Verification items for the finished model (mm, model axes). Face numbers are marked on the shaded views. A direction names the side the tool comes from. Coordinates: 2 decimals unless noted, no trailing zeros. Order: outer loops, then holes, each group sorted by start corner. A loop starts at its lowest first (then second) coordinate and runs counter-clockwise, first axis right, second up. Notation, with made-up numbers: (-37.5, 69.5) -> (-27.5, 69.5) arc R26 ccw to (-27.5, 104.5) -> close; hole circle Ø8 at (57.25, -33). An arc over 180 degrees is marked (long way). Write each question's results on one line, items separated by ' | '. Start each with the question number.
(1) Go/stop test with flat-tipped pins: pin 1 (5 mm diameter, centred on x = 16.16, y = 28, fed in from +Z); pin 2 (11.5 mm diameter, centred on x = -35.5, y = -2, fed in from +Z); pin 3 (9 mm diameter, centred on y = 9.5, z = 20.5, fed in from -X); pin 4 (1 mm diameter, centred on x = -15.5, y = 27.5, fed in from -Z). Record where each tip stops, or that it passes through.
(2) Draft check along X on the marked faces 5, 6, 7 and 8. Enter one of: +X half, -X half, draft (parallel to the pull), parting line (faces both ways), or undercut.
(3) Cross-section at C-C on z = 26.5. Enter the section's corners in (x, y), and give its area (3 significant figures).
(4) Thickness scan on probe 1 along X at (y, z) = (0, 6.75); probe 2 along X at (y, z) = (0, 11.95); probe 3 along Y at (x, z) = (-3, 22). Record the ranges inside material, lowest first. Write a range as [from, to].
(5) Cross-section at A-A on x = 0. Enter the section's corners in (y, z).
(6) Cross-section at D-D on x = -10. Give the number of separate pieces and of enclosed holes in the cut face, and give its area (3 significant figures).
(7) Cross-section at B-B on z = 22. Enter the section's corners in (x, y), and give its area (3 significant figures).
(8) Set-up check for the marked faces 1, 2, 3 and 4: record each of +Z, -Z, +X, -X, +Y, -Y from which the full face is reachable in a straight line by a thin tool's end or side.
```python
from build123d import *

# Parameters (mm, degrees)
SKETCH1_R                                     = 39.5
SKETCH1_R_2                                   = 28.5
BOSS_EXTRUDE1_DEPTH                           = 11
SKETCH2_R                                     = 39.5
BOSS_EXTRUDE2_DEPTH                           = 20
CUT_EXTRUDE3_START                            = -27
CUT_EXTRUDE3_DEPTH                            = 27
CUT_EXTRUDE4_START                            = -18
CUT_EXTRUDE4_DEPTH                            = 18
CBORE_FOR_M3_HEX_HEAD_MACHINE_SCREW1_AT_COUNT = 2
CBORE_FOR_M3_HEX_HEAD_MACHINE_SCREW1_AT_PITCH = 68
CBORE_FOR_M3_HEX_HEAD_MACHINE_SCREW1_2_COUNT  = 2
CBORE_FOR_M3_HEX_HEAD_MACHINE_SCREW1_2_PITCH  = 58.889727457
CBORE_FOR_M3_HEX_HEAD_MACHINE_SCREW1_3_COUNT  = 2
CBORE_FOR_M3_HEX_HEAD_MACHINE_SCREW1_3_PITCH  = 34
FILLET2_R                                     = 2
CBORE_FOR_M3_HEX_HEAD_MACHINE_SCREW2_AT_COUNT = 2
CBORE_FOR_M3_HEX_HEAD_MACHINE_SCREW2_AT_PITCH = 32.326095378
CUT_EXTRUDE5_DEPTH                            = 82.740442866
CUT_EXTRUDE5_DEPTH_BACK                       = 82.740442866
SKETCH10_R                                    = 2
FILLET5_R                                     = 5
FILLET4_R                                     = 5
FILLET6_R                                     = 1
FILLET7_R                                     = 10


with BuildPart() as part:
    # Sketch1 → Boss-Extrude1 (new body)
    with BuildSketch(Plane.XY):
        Circle(SKETCH1_R)
        Circle(SKETCH1_R_2, mode=Mode.SUBTRACT)
    extrude(amount=BOSS_EXTRUDE1_DEPTH)

    # Sketch2 → Boss-Extrude2 (add)
    with BuildSketch(Plane.XY.offset(11)):
        Circle(SKETCH2_R)
    extrude(amount=BOSS_EXTRUDE2_DEPTH)

    # Sketch3 → Cut-Extrude3 (cut)
    with BuildSketch(Plane.XY.offset(31).offset(CUT_EXTRUDE3_START)):
        with BuildLine():
            ThreePointArc((-32.806249405, -22), (0, -39.5), (32.806249405, -22))
            Line((32.806249405, -22), (-32.806249405, -22))
        make_face()
    extrude(amount=CUT_EXTRUDE3_DEPTH, mode=Mode.SUBTRACT)

    # Sketch4 → Cut-Extrude4 (cut)
    with BuildSketch(Plane.XY.offset(31).offset(CUT_EXTRUDE4_START)):
        with BuildLine():
            Line((-32.806249405, -22), (-25, -22))
            Line((-25, -22), (-25, 30.581857367))
            ThreePointArc((-25, 30.581857367), (-39.071774321, 5.800556129), (-32.806249405, -22))
        make_face()
        with BuildLine():
            Line((25, 30.581857367), (25, -22))
            Line((25, -22), (32.806249405, -22))
            ThreePointArc((32.806249405, -22), (39.071774321, 5.800556129), (25, 30.581857367))
        make_face()
    extrude(amount=CUT_EXTRUDE4_DEPTH, mode=Mode.SUBTRACT)

    # Sketch6 → CBORE for M3 Hex Head Machine Screw1 (revolve, cut)
    with BuildSketch(Plane(origin=(-34, 0, 13), x_dir=(0, -1, 0), z_dir=(1, 0, 0))):
        Polygon((0, 0), (0, 13), (1.7, 13), (1.7, 2.3), (4.2, 2.3), (4.2, 0.025), (4.225, 0), align=None)
    cbore_for_m3_hex_head_machine_screw1 = revolve(axis=Axis((-34, 0, 19.35), (0, 0, -1)), mode=Mode.SUBTRACT)

    # CBORE for M3 Hex Head Machine Screw1 at: CBORE for M3 Hex Head Machine Screw1 ×2
    with Locations(*[(i * CBORE_FOR_M3_HEX_HEAD_MACHINE_SCREW1_AT_PITCH, 0, 0) for i in range(1, CBORE_FOR_M3_HEX_HEAD_MACHINE_SCREW1_AT_COUNT)]):
        add(cbore_for_m3_hex_head_machine_screw1, mode=Mode.SUBTRACT)

    # CBORE for M3 Hex Head Machine Screw1 2: CBORE for M3 Hex Head Machine Screw1 ×2
    with Locations(*[Vector(0.8660254037844364, -0.500000000000004, 0) * (i * CBORE_FOR_M3_HEX_HEAD_MACHINE_SCREW1_2_PITCH) for i in range(1, CBORE_FOR_M3_HEX_HEAD_MACHINE_SCREW1_2_COUNT)]):
        add(cbore_for_m3_hex_head_machine_screw1, mode=Mode.SUBTRACT)

    # CBORE for M3 Hex Head Machine Screw1 3: CBORE for M3 Hex Head Machine Screw1 ×2
    with Locations(*[Vector(0.4999999999999949, -0.8660254037844417, 0) * (i * CBORE_FOR_M3_HEX_HEAD_MACHINE_SCREW1_3_PITCH) for i in range(1, CBORE_FOR_M3_HEX_HEAD_MACHINE_SCREW1_3_COUNT)]):
        add(cbore_for_m3_hex_head_machine_screw1, mode=Mode.SUBTRACT)

    # Fillet2
    fillet2_edges = [part.edges().sort_by_distance(p)[0] for p in [
        (-18.117670932, -22, 7.5),
        (18.117670932, -22, 7.5),
    ]]
    fillet(fillet2_edges, radius=FILLET2_R)

    # Sketch8 → CBORE for M3 Hex Head Machine Screw2 (revolve, cut)
    with BuildSketch(Plane(origin=(-16.163047689, 27.995219802, 31), x_dir=(0, -1, 0), z_dir=(1, 0, 0))):
        Polygon((0, 0), (0, 31), (1.7, 31), (1.7, 2.3), (4.2, 2.3), (4.2, 0.025), (4.225, 0), align=None)
    cbore_for_m3_hex_head_machine_screw2 = revolve(axis=Axis((-16.163047689, 27.995219802, 37.35), (0, 0, -1)), mode=Mode.SUBTRACT)

    # CBORE for M3 Hex Head Machine Screw2 at: CBORE for M3 Hex Head Machine Screw2 ×2
    with Locations(*[(i * CBORE_FOR_M3_HEX_HEAD_MACHINE_SCREW2_AT_PITCH, 0, 0) for i in range(1, CBORE_FOR_M3_HEX_HEAD_MACHINE_SCREW2_AT_COUNT)]):
        add(cbore_for_m3_hex_head_machine_screw2, mode=Mode.SUBTRACT)

    # Sketch10 → Cut-Extrude5 (cut, two sides: drawn at the far end of the back side and taken through both)
    with BuildSketch(Plane.ZY.offset(25).offset(-CUT_EXTRUDE5_DEPTH_BACK)):
        with Locations(Location((22, 20, 0), (0, 0, 180))):
            Circle(SKETCH10_R)
        with Locations(Location((22, -15, 0), (0, 0, 180))):
            Circle(SKETCH10_R)
    extrude(amount=CUT_EXTRUDE5_DEPTH + CUT_EXTRUDE5_DEPTH_BACK, mode=Mode.SUBTRACT)

    # Fillet5
    fillet5_edges = [part.edges().sort_by_distance(p)[0] for p in [
        (32.806249405, -22, 8.5),
        (-32.806249405, -22, 8.5),
    ]]
    fillet(fillet5_edges, radius=FILLET5_R)

    # Fillet4
    # the kernel refuses this fillet: 5 mm, written as the material it adds along each edge
    with BuildSketch(Plane(origin=(-23.027157879, -22, 4), x_dir=(0, 0, 1), z_dir=(-1, 0, 0))) as fillet4_piece_1_section:
        with BuildLine():
            CenterArc((FILLET4_R, -FILLET4_R), FILLET4_R, 90, 90)
            Line((0, -FILLET4_R), (0, 0))
            Line((0, 0), (FILLET4_R, 0))
        make_face()
    fillet4_piece_1 = extrude(amount=6.993668225, mode=Mode.PRIVATE)
    fillet4_piece_1 = fillet4_piece_1 & Plane(origin=(0, 0, 5.117497097), x_dir=(1, 0, 0), z_dir=(0, 0, -1)) * Cylinder(39.5, 34, mode=Mode.PRIVATE)
    add(fillet4_piece_1)
    with BuildSketch(Plane(origin=(30.020826105, -17, 4), x_dir=(0, -1, 0), z_dir=(-1, 0, 0))) as fillet4_piece_2_section:
        with BuildLine():
            CenterArc((5 + FILLET4_R, FILLET4_R), FILLET4_R, 180, 90)
            Line((5 + FILLET4_R, 0), (5, 0))
            Line((5, 0), (5, FILLET4_R))
        make_face()
    fillet4_piece_2 = revolve(axis=Axis((30.020826105, -17, 4), (0, 0, 1)), revolution_arc=203.743697153, mode=Mode.PRIVATE)
    fillet4_piece_2 = fillet4_piece_2 - Plane(origin=(0, 0, 5.881838576), x_dir=(1, 0, 0), z_dir=(0, 0, -1)) * Cylinder(28.5, 40, mode=Mode.PRIVATE)
    fillet4_piece_2 = fillet4_piece_2 & Plane(origin=(0, 0, 5.881838576), x_dir=(1, 0, 0), z_dir=(0, 0, -1)) * Cylinder(39.5, 40, mode=Mode.PRIVATE)
    add(fillet4_piece_2)
    with BuildSketch(Plane(origin=(-30.020826105, -17, 4), x_dir=(0, -1, 0), z_dir=(1, 0, 0))) as fillet4_piece_3_section:
        with BuildLine():
            CenterArc((5 + FILLET4_R, -FILLET4_R), FILLET4_R, 90, 90)
            Line((5 + FILLET4_R, 0), (5, 0))
            Line((5, 0), (5, -FILLET4_R))
        make_face()
    fillet4_piece_3 = revolve(axis=Axis((-30.020826105, -17, 4), (0, 0, -1)), revolution_arc=203.743697153, mode=Mode.PRIVATE)
    fillet4_piece_3 = fillet4_piece_3 - Plane(origin=(0, 0, 5.881838618), x_dir=(1, 0, 0), z_dir=(0, 0, -1)) * Cylinder(28.5, 40, mode=Mode.PRIVATE)
    fillet4_piece_3 = fillet4_piece_3 & Plane(origin=(0, 0, 5.881838618), x_dir=(1, 0, 0), z_dir=(0, 0, -1)) * Cylinder(39.5, 40, mode=Mode.PRIVATE)
    add(fillet4_piece_3)
    with BuildSketch(Plane(origin=(30.020826105, -22, 4), x_dir=(0, 0, 1), z_dir=(-1, 0, 0))) as fillet4_piece_4_section:
        with BuildLine():
            CenterArc((FILLET4_R, -FILLET4_R), FILLET4_R, 90, 90)
            Line((0, -FILLET4_R), (0, 0))
            Line((0, 0), (FILLET4_R, 0))
        make_face()
    fillet4_piece_4 = extrude(amount=6.993668225, mode=Mode.PRIVATE)
    fillet4_piece_4 = fillet4_piece_4 & Plane(origin=(0, 0, 5.117497097), x_dir=(1, 0, 0), z_dir=(0, 0, -1)) * Cylinder(39.5, 34, mode=Mode.PRIVATE)
    add(fillet4_piece_4)
    with BuildSketch(Plane(origin=(-23.027157879, -20, 4), x_dir=(0, -1, 0), z_dir=(-1, 0, 0))) as fillet4_piece_5_section:
        with BuildLine():
            CenterArc((2 + FILLET4_R, FILLET4_R), FILLET4_R, 180, 90)
            Line((2 + FILLET4_R, 0), (2, 0))
            Line((2, 0), (2, FILLET4_R))
        make_face()
    fillet4_piece_5 = revolve(axis=Axis((-23.027157879, -20, 4), (0, 0, 1)), revolution_arc=359.64, mode=Mode.PRIVATE)
    fillet4_piece_5 = fillet4_piece_5 - Plane(origin=(0, 0, 5.416079677), x_dir=(1, 0, 0), z_dir=(0, 0, -1)) * Cylinder(28.5, 28, mode=Mode.PRIVATE)
    add(fillet4_piece_5)
    with BuildSketch(Plane(origin=(23.027157879, -20, 4), x_dir=(0, -1, 0), z_dir=(1, 0, 0))) as fillet4_piece_6_section:
        with BuildLine():
            CenterArc((2 + FILLET4_R, -FILLET4_R), FILLET4_R, 90, 90)
            Line((2 + FILLET4_R, 0), (2, 0))
            Line((2, 0), (2, -FILLET4_R))
        make_face()
    fillet4_piece_6 = revolve(axis=Axis((23.027157879, -20, 4), (0, 0, -1)), revolution_arc=359.64, mode=Mode.PRIVATE)
    fillet4_piece_6 = fillet4_piece_6 - Plane(origin=(0, 0, 5.416079623), x_dir=(1, 0, 0), z_dir=(0, 0, -1)) * Cylinder(28.5, 28, mode=Mode.PRIVATE)
    add(fillet4_piece_6)

    # Fillet6
    # the kernel refuses this fillet: 1 mm, written as the material it adds along each edge
    with BuildSketch(Plane(origin=(0, 0, 11), x_dir=(1, 0, 0), z_dir=(0, -1, 0))) as fillet6_piece_1:
        with BuildLine():
            CenterArc((28.5 - FILLET6_R, -FILLET6_R), FILLET6_R, 0, 90)
            Line((28.5 - FILLET6_R, 0), (28.5, 0))
            Line((28.5, 0), (28.5, -FILLET6_R))
        make_face()
    revolve(axis=Axis((0, 0, 11), (0, 0, 1)), revolution_arc=220.975610343)
    with BuildSketch(Plane(origin=(-23.027157879, -20, 11), x_dir=(-0.9493195168959316, -0.31431267050578, 0), z_dir=(-0.31431267050578, 0.9493195168959316, 0))) as fillet6_piece_2_section:
        with BuildLine():
            CenterArc((2 + FILLET6_R, -FILLET6_R), FILLET6_R, 90, 90)
            Line((2, -FILLET6_R), (2, 0))
            Line((2, 0), (2 + FILLET6_R, 0))
        make_face()
    fillet6_piece_2 = revolve(axis=Axis((-23.027157879, -20, 11), (0, 0, 1)), revolution_arc=202.656285008, mode=Mode.PRIVATE)
    fillet6_piece_2 = split(fillet6_piece_2, bisect_by=Plane(origin=(-21.199330991, -22, 10.4999997), z_dir=(0, 1, 0)), keep=Keep.TOP, mode=Mode.PRIVATE)
    add(fillet6_piece_2)
    with BuildSketch(Plane(origin=(23.027157879, -20, 11), x_dir=(0.9493195168959316, -0.31431267050578, 0), z_dir=(0.31431267050578, 0.9493195168959316, 0))) as fillet6_piece_3_section:
        with BuildLine():
            CenterArc((2 + FILLET6_R, FILLET6_R), FILLET6_R, 180, 90)
            Line((2 + FILLET6_R, 0), (2, 0))
            Line((2, 0), (2, FILLET6_R))
        make_face()
    fillet6_piece_3 = revolve(axis=Axis((23.027157879, -20, 11), (0, 0, -1)), revolution_arc=202.656285008, mode=Mode.PRIVATE)
    fillet6_piece_3 = split(fillet6_piece_3, bisect_by=Plane(origin=(20.946630344, -22, 10.713386851), z_dir=(0, 1, 0)), keep=Keep.TOP, mode=Mode.PRIVATE)
    add(fillet6_piece_3)
    with BuildSketch(Plane(origin=(0, 0, 11), x_dir=(0.7549887829291444, -0.6557377049180327, 0), z_dir=(-0.6557377049180327, -0.7549887829291444, 0))) as fillet6_piece_4:
        with BuildLine():
            CenterArc((28.5 - FILLET6_R, -FILLET6_R), FILLET6_R, 0, 90)
            Line((28.5 - FILLET6_R, 0), (28.5, 0))
            Line((28.5, 0), (28.5, -FILLET6_R))
        make_face()
    revolve(axis=Axis((0, 0, 11), (0, 0, 1)), revolution_arc=40.975610343)

    # Fillet7
    fillet7_edges = [part.edges().sort_by_distance(p)[0] for p in [
        (0, -22, 31),
    ]]
    fillet(fillet7_edges, radius=FILLET7_R)


solid = part.part
```
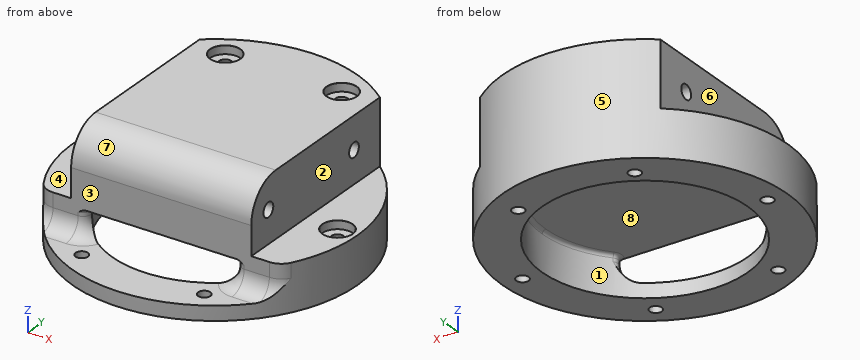
Results are:
1) pin 1: stops at z = 28.7 | pin 2: stops at z = 13 | pin 3: stops at x = -25 | pin 4: passes through
2) face 5: parting line | face 6: -X half | face 7: draft | face 8: undercut
3) outline: (-25, -20.35) -> (25, -20.35) -> (25, 30.58) arc R39.5 ccw to (-25, 30.58) -> close; hole circle Ø3.4 at (-16.16, 28); hole circle Ø3.4 at (16.16, 28) | area: 2,830 mm2
4) probe 1: x = [-39.5, -35.7], [-32.3, -28.5], [28.5, 32.3], [35.7, 39.5] | probe 2: x = [-39.5, -38.2], [-29.8, 29.8], [38.2, 39.5] | probe 3: y = [-21.95, -17], [-13, 18], [22, 39.39]
5) outline: (-39.5, 0) -> (-28.5, 0) -> (-28.5, 4) -> (-39.5, 4) -> close; (-22, 11) -> (27.5, 11) arc R1 cw to (28.5, 10) -> (28.5, 0) -> (39.5, 0) -> (39.5, 31) -> (-12, 31) arc R10 ccw to (-22, 21) -> close; hole circle Ø4 at (-15, 22); hole circle Ø4 at (20, 22)
6) separate pieces: 2 | enclosed holes: 2 | area: 1,330 mm2
7) outline: (-25, -21.95) -> (25, -21.95) -> (25, -17) -> (-25, -17) -> close; (-25, -13) -> (25, -13) -> (25, 18) -> (-25, 18) -> close; (-25, 22) -> (25, 22) -> (25, 30.58) arc R39.5 ccw to (-25, 30.58) -> close; hole circle Ø3.4 at (-16.16, 28); hole circle Ø3.4 at (16.16, 28) | area: 2,510 mm2
8) face 1: -Z | face 2: +Z, +X, +Y, -Y | face 3: +Z, +X, -X, -Y | face 4: +Z, -X, +Y, -Y
